from build123d import *
from OCP.BRepFilletAPI import BRepFilletAPI_MakeChamfer

# Parameters (mm, degrees)
SKETCH1_R           = 7
BOSS_EXTRUDE1_DEPTH = 10
SKETCH1_5_W         = 30
SKETCH1_5_H         = 30
SKETCH1_5_R         = 7
BOSS_EXTRUDE2_DEPTH = 40
SKETCH1_11_W        = 5
SKETCH1_11_H        = 14
BOSS_EXTRUDE5_DEPTH = 15
BOSS_EXTRUDE6_DEPTH = 15
BOSS_EXTRUDE7_DEPTH = 40
CHAMFER2_SIZE       = 30
CHAMFER2_SIZE2      = 10
SKETCH4_W           = 5
SKETCH4_H           = 14
CUT_EXTRUDE3_DEPTH  = 74.409808609


with BuildPart() as part:
    # Sketch1 → Boss-Extrude1 (new body)
    with BuildSketch(Plane(origin=(0, 0, 0), x_dir=(1, 0, 0), z_dir=(0, 1, 0))):
        with BuildLine():
            Line((-15, 0), (-15, 12))
            Line((-15, 12), (15, 12))
            Line((15, 12), (15, 0))
            ThreePointArc((15, 0), (0, -15), (-15, 0))
        make_face()
        with Locations(Location((0, 0, 0), (0, 0, 270))):
            Circle(SKETCH1_R, mode=Mode.SUBTRACT)
    extrude(amount=BOSS_EXTRUDE1_DEPTH)

    # Sketch1_5 → Boss-Extrude2 (add)
    with BuildSketch(Plane(origin=(0, 0, 0), x_dir=(1, 0, 0), z_dir=(0, 1, 0))):
        with Locations((0, 27)):
            Rectangle(SKETCH1_5_W, SKETCH1_5_H)
        with Locations(Location((0, 27, 0), (0, 0, 270))):
            Circle(SKETCH1_5_R, mode=Mode.SUBTRACT)
    extrude(amount=BOSS_EXTRUDE2_DEPTH)



with BuildPart() as body_2:
    # Sketch1_11 → Boss-Extrude5 (new body)
    with BuildSketch(Plane(origin=(0, 0, 0), x_dir=(1, 0, 0), z_dir=(0, 1, 0))):
        Polygon((45, 42), (25, 42), (25, 34), (40, 34), (45, 34), align=None)
        with Locations((42.5, 27)):
            Rectangle(SKETCH1_11_W, SKETCH1_11_H)
        Polygon((25, 20), (25, 12), (45, 12), (45, 20), (40, 20), align=None)
    extrude(amount=BOSS_EXTRUDE5_DEPTH)


with BuildPart() as body_3:
    # Sketch1_12 → Boss-Extrude6 (new body)
    with BuildSketch(Plane(origin=(0, 0, 0), x_dir=(1, 0, 0), z_dir=(0, 1, 0))):
        Polygon((-45, 12), (-25, 12), (-25, 20), (-40, 20), (-40, 34), (-25, 34), (-25, 42), (-45, 42), align=None)
    extrude(amount=BOSS_EXTRUDE6_DEPTH)


with BuildPart() as part_1:
    add(part.part)

    add(body_2.part)  # Boss-Extrude7 merges body 2

    add(body_3.part)  # Boss-Extrude7 merges body 3
    # Sketch1_13 → Boss-Extrude7 (add)
    with BuildSketch(Plane(origin=(0, 0, 0), x_dir=(1, 0, 0), z_dir=(0, 1, 0))):
        Polygon((-25, 12), (-15, 12), (-15, 42), (-25, 42), (-25, 34), (-25, 20), align=None)
        Polygon((15, 42), (15, 12), (25, 12), (25, 20), (25, 34), (25, 42), align=None)
    extrude(amount=BOSS_EXTRUDE7_DEPTH)

    # Chamfer2: one chamfer whose edges measure the first distance from different faces: ONE call of the kernel's chamfer builder (chamfer() names one face for all edges)
    chamfer2_edges_1 = [part_1.edges().sort_by_distance(p)[0] for p in [
        (25, 40, -27),
    ]]
    chamfer2_side_1 = [part_1.faces().sort_by_distance(p)[0] for p in [
        (25, 23.125, -27),
    ]]
    chamfer2_edges_2 = [part_1.edges().sort_by_distance(p)[0] for p in [
        (-25, 40, -27),
    ]]
    chamfer2_side_2 = [part_1.faces().sort_by_distance(p)[0] for p in [
        (-25, 23.125, -27),
    ]]
    chamfer2 = BRepFilletAPI_MakeChamfer(part_1.part.solid().wrapped)
    for e in chamfer2_edges_1:
        chamfer2.Add(CHAMFER2_SIZE, CHAMFER2_SIZE2, e.wrapped, chamfer2_side_1[0].wrapped)  # the first distance lies on this face
    for e in chamfer2_edges_2:
        chamfer2.Add(CHAMFER2_SIZE, CHAMFER2_SIZE2, e.wrapped, chamfer2_side_2[0].wrapped)  # the first distance lies on this face
    add(Compound.cast(chamfer2.Shape()), mode=Mode.REPLACE)

    # Sketch4 → Cut-Extrude3 (cut, through all)
    with BuildSketch(Plane.XZ):
        with Locations((-22.5, -27)):
            Rectangle(SKETCH4_W, SKETCH4_H)
        with Locations((22.5, -27)):
            Rectangle(SKETCH4_W, SKETCH4_H)
    extrude(amount=-CUT_EXTRUDE3_DEPTH, mode=Mode.SUBTRACT)


solid = part_1.part
Part model, mm, in its own coordinate system. A direction names the side the tool comes from. Round coordinates to 2 decimals unless told otherwise and drop trailing zeros. Write each loop counter-clockwise with the first axis right and the second up, starting at its lowest first coordinate (ties: lowest second). Pieces come first, ordered by that corner, then holes. Notation, with made-up numbers: M 5.25,-25.75 L 55.25,-25.75 A29 ccw 55.25,11.25 Z; hole C 86,41 d9. An arc over 180 degrees is marked long. Return JSON: item names as keys, results as strings. Group by question number.
(1) Two-plate mould, pull along X, no slides. Class faces 1 (the face through (41, 15, -27)), 2 (the face through (0, 5, 15)), 3 (the face through (30, 7, -34)), 4 (the face through (-30, 7, -20)): +X half, -X half, draft (parallel to the pull), parting line (faces both ways), or undercut.
(2) Pin check, flat tips, straight feed: pin 1 Ø10 at (y, z) = (34.5, -31) entering from +X; pin 2 Ø17.5 at (x, z) = (-35.5, -21) entering from +Y; pin 3 Ø5 at (y, z) = (3, -7) entering from +X. Stop position of each tip, or through.
(3) Drill centre lines: probe 1 along X at (y, z) = (5.5, -24); probe 2 along Z at (x, y) = (0.5, 18); probe 3 along Y at (x, z) = (-26.5, -18). Where is each one in solid material? Low to high.
(4) Saw through at A-A on x = 0. Write the cut outline in (y, z).
(5) Saw through at D-D on y = 29.5. Write the cut outline in (x, z).
(6) Which spindle directions (+Z, -Z, +X, -X, +Y, -Y) get a long thin tool onto all of the face, cutting with end or side? Do faces 5 (the face through (-15, 5, -6)), 6 (the face through (-42, 15, -27)), 7 (the face through (15, 5, -6)), 8 (the face through (-30, 7, -34)). Say none if no direction does.
(7) Saw through at C-C on x = -25.5. Write the cut outline in (y, z).
(8) Saw through at B-B on z = 3.5. Write the cut outline in (x, y).
Returned:
{
 "1": {"face 1": "draft", "face 2": "parting line", "face 3": "undercut", "face 4": "undercut"},
 "2": {"pin 1": "x = 18.5", "pin 2": "y = 15", "pin 3": "x = 15"},
 "3": {"probe 1": "-45 to -40, -20 to -6.32, 6.32 to 20, 40 to 45", "probe 2": "-42 to -33.98, -20.02 to -12", "probe 3": "0 to 15"},
 "4": {"outline": "M 0,-42 L 40,-42 L 40,-34 L 0,-34 Z; M 0,-20 L 40,-20 L 40,-12 L 10,-12 L 10,-7 L 0,-7 Z; M 0,7 L 10,7 L 10,15 L 0,15 Z"},
 "5": {"outline": "M -18.5,-42 L 18.5,-42 L 18.5,-12 L -18.5,-12 Z; hole C 0,-27 d14"},
 "6": {"face 5": "+Z, -X, +Y, -Y", "face 6": "+Z, -Z, -X, +Y", "face 7": "+Z, +X, +Y, -Y", "face 8": "+Y, -Y"},
 "7": {"outline": "M 0,-42 L 15,-42 L 15,-34 L 0,-34 Z; M 0,-20 L 15,-20 L 15,-12 L 0,-12 Z"},
 "8": {"outline": "M -14.59,0 L -6.06,0 L -6.06,10 L -14.59,10 Z; M 6.06,0 L 14.59,0 L 14.59,10 L 6.06,10 Z"}
}
